Autodesk Inventor part; units mm, degrees
ref_plane "YZ Plane" through (0, 0, 0) normal (1, 0, 0) x (0, 1, 0)
ref_plane "XZ Plane" through (0, 0, 0) normal (0, 1, 0) x (-1, 0, 0)
ref_plane "XY Plane" through (0, 0, 0) normal (0, 0, 1) x (1, 0, 0)
sketch "Sketch2" plane through (0, 0, 0) normal (0, 0, 1) x (1, 0, 0)
  line L0 (7.62, 0) -> (3.81, -6.5991)
  line L1 (3.81, -6.5991) -> (-3.81, -6.5991)
  line L2 (-3.81, -6.5991) -> (-7.62, 0)
  line L3 (-7.62, 0) -> (-3.81, 6.5991)
  line L4 (-3.81, 6.5991) -> (3.81, 6.5991)
  line L5 (3.81, 6.5991) -> (7.62, 0)
  line L6 (25.4, 0) -> (12.7, -21.997)
  line L7 (12.7, -21.997) -> (-12.7, -21.997)
  line L8 (-12.7, -21.997) -> (-25.4, 0)
  line L9 (-25.4, 0) -> (-12.7, 21.997)
  line L10 (-12.7, 21.997) -> (12.7, 21.997)
  line L11 (12.7, 21.997) -> (25.4, 0)
  point P0 (0, 0)
  point P1 (0, 0)
  point P2 (0, 0)
  dimension "d2" = 7.62
  dimension "d3" = 25.4
extrude "Extrusion1" add sketch "Sketch2" along normal blind 76.2
properties part number "HexSpacer"
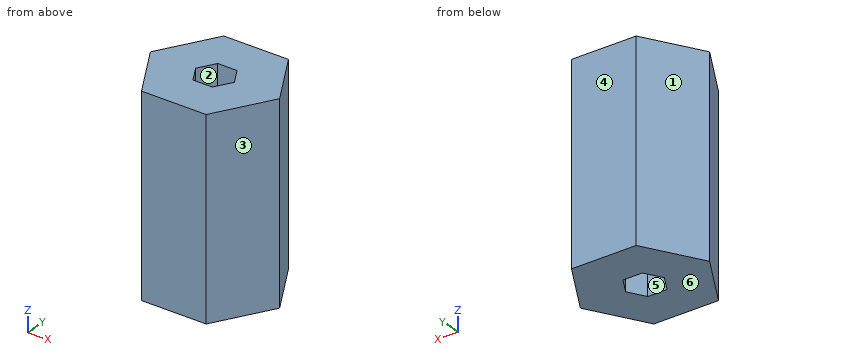
The model under review builds one solid part; all positions refer to its coordinate system, in mm. Face numbers are marked on the shaded views. A direction names the side the tool comes from. Give positions to 0.01 mm unless a question says otherwise; leave off trailing zeros. Write each loop counter-clockwise with the first axis right and the second up, starting at its lowest first coordinate (ties: lowest second). Pieces come first, ordered by that corner, then holes. Notation, with made-up numbers: M 7,81 L 40,81 A10 cw 40,100 Z; hole C -14,39.5 d2. An arc over 180 degrees is marked long. Write each question's results on one line, items separated by ' | '. Start each with the question number.
1. Insertion check: pin 1 Ø3 at (y, z) = (7, 50) entering from -X; pin 2 Ø5 at (x, y) = (-12.5, -6.5) entering from -Z. Each pin has a flat end and moves straight along its axis. Give the tip position at first contact, or say it passes through.
2. We need section D-D (y = 15). Write out the cut boundary in (x, z), and give its area (3 significant figures).
3. We need section C-C (x = -22). Write out the cut boundary in (y, z).
4. We need section B-B (y = -4). Write out the cut boundary in (x, z).
5. For the marked faces 5 and 6, list the 3-axis set-ups (+Z, -Z, +X, -X, +Y, -Y) from which the entire face can be reached by the end or side of a thin tool; tool diameter is ignored.
6. We need section A-A (z = 28). Write out the cut boundary in (x, y).
7. For probe 1 along Y at (x, z) = (-3, 66); probe 2 along X at (y, z) = (-1, 59.5); probe 3 along X at (y, z) = (-5, 50), list the stretches that pass through material, from the lowest coordinate up. Write a range as [from, to].
8. Mouldability with a two-part tool opening along X and no side actions: class the marked faces 1, 2, 3 and 4 as released by +X, released by -X, zero draft, split by the parting line, or undercut.
Results found:
1) pin 1: stops at x = -22.22 | pin 2: stops at z = 0
2) outline: M -16.74,0 L 16.74,0 L 16.74,76.2 L -16.74,76.2 Z | area: 2,550 mm^2
3) outline: M -5.89,0 L 5.89,0 L 5.89,76.2 L -5.89,76.2 Z
4) outline: M -23.09,0 L -5.31,0 L -5.31,76.2 L -23.09,76.2 Z; M 5.31,0 L 23.09,0 L 23.09,76.2 L 5.31,76.2 Z
5) face 5: +Z, -Z | face 6: -Z, +X, -X, +Y, -Y
6) outline: M -25.4,0 L -12.7,-22 L 12.7,-22 L 25.4,0 L 12.7,22 L -12.7,22 Z; hole M -7.62,0 L -3.81,-6.6 L 3.81,-6.6 L 7.62,0 L 3.81,6.6 L -3.81,6.6 Z
7) probe 1: y = [-22, -6.6], [6.6, 22] | probe 2: x = [-24.82, -7.04], [7.04, 24.82] | probe 3: x = [-22.51, -4.73], [4.73, 22.51]
8) face 1: released by -X | face 2: undercut | face 3: released by +X | face 4: zero draft
